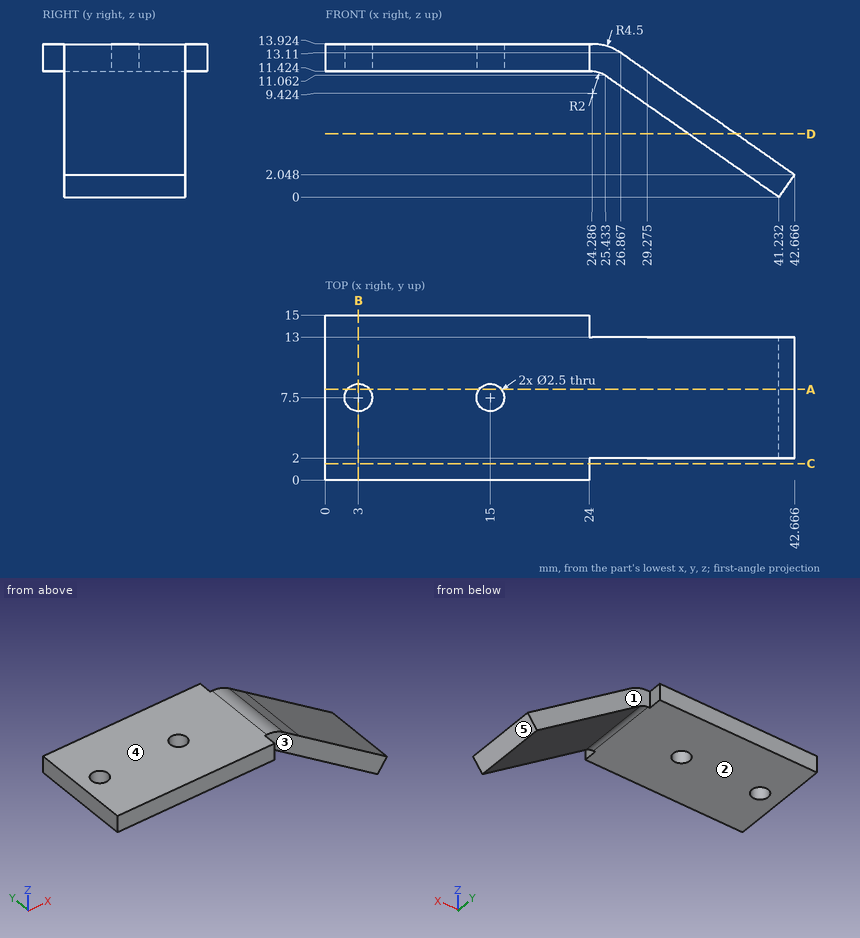
Geometry: see drawing. Coordinates: mm, zero at the bounding-box minimum. A direction names the side the tool comes from. Coordinates: 2 decimals unless noted, no trailing zeros. Loops run counter-clockwise (first coordinate to the right, second up) from the corner with the lowest first, then second, coordinate; pieces in that order, holes last.
Q1. Contact query for flat-ended pins moving along their axis: pin 1 (6 mm diameter, centred on x = 38, z = 2.5, fed in from -Y); pin 2 (6 mm diameter, centred on y = 2, z = 6.5, fed in from -X) (1 decimal); pin 3 (0.6 mm diameter, centred on y = 1.5, z = 12, fed in from +X). Output: stop coordinate, or through.
Q2. Cut plane C-C (y = 1.5). Output: boundary loops of the cut face in (x, z).
Q3. Cut plane A-A (y = 8.25). Output: boundary loops of the cut face in (x, z) (1 decimal).
Q4. Set-up query: the marked faces 1, 2, 3, 4 and 5. Return all of +Z, -Z, +X, -X, +Y, -Y with unobstructed straight access to the full face (end or side cutting, diameter ignored); none if empty.
Q5. Cut plane B-B (x = 3). Output: boundary loops of the cut face in (y, z).
Q6. Cut plane D-D (z = 5.75). Output: boundary loops of the cut face in (x, y).
Q7. Material intervals for line 1 (Y direction, x = 15, z = 12.7); line 2 (Z direction, x = 18.5, y = 10.25); line 3 (X direction, y = 8, z = 11.5) (1 decimal), sorted ascending.
Working result:
1. pin 1: stops at y = 2
1. pin 2: stops at x = 27.7
1. pin 3: stops at x = 24
2. outline: (0, 11.42) - (24, 11.42) - (24, 13.92) - (0, 13.92) - close
3. outline: (0, 11.4) - (2, 11.4) - (2, 13.9) - (0, 13.9) - close; (4, 11.4) - (14, 11.4) - (14, 13.9) - (4, 13.9) - close; (16, 11.4) - (24.3, 11.4) arc R2 cw to (25.4, 11.1) - (41.2, 0) - (42.7, 2) - (26.9, 13.1) arc R4.5 ccw to (24.3, 13.9) - (16, 13.9) - close
4. face 1: +Z, -Z, +X, +Y
4. face 2: -Z, -X, +Y, -Y
4. face 3: +Z, -Z, +X, -Y
4. face 4: +Z, +X, -X, +Y, -Y
4. face 5: -Z, +X, +Y, -Y
5. outline: (0, 11.42) - (6.25, 11.42) - (6.25, 13.92) - (0, 13.92) - close; (8.75, 11.42) - (15, 11.42) - (15, 13.92) - (8.75, 13.92) - close
6. outline: (33.02, 2) - (37.38, 2) - (37.38, 13) - (33.02, 13) - close
7. line 1: y = 0 to 6.25, 8.75 to 15
7. line 2: z = 11.42 to 13.92
7. line 3: x = 0 to 1.9, 4.1 to 13.9, 16.1 to 29.2
